from build123d import *

# Parameters (mm, degrees)
BOSS_EXTRUDE1_DEPTH     = 19.05
F_1_4_CLEARANCE_HOLE1_D = 6.5278
F_10_32_TAPPED_HOLE1_D  = 4.0386
SKETCH6_R               = 1.5875
CUT_EXTRUDE1_DEPTH      = 52.373383773
LPATTERN1_COUNT         = 9
LPATTERN1_PITCH         = 5.00126
FILLET1_R               = 3.429


with BuildPart() as part:
    # Sketch1 → Boss-Extrude1 (new body)
    with BuildSketch(Plane.XY):
        Polygon((0, 0), (17.3355, 0), (17.3355, 44.45), (0, 44.45), (0, 28.575), (9.525, 28.575), (9.525, 15.875), (0, 15.875), align=None)
    extrude(amount=BOSS_EXTRUDE1_DEPTH)

    # 1/4 Clearance Hole1 (through all)
    with Locations(Plane.XY.offset(19.05)):
        with Locations((5.842, 38.1), (5.842, 6.35)):
            Hole(F_1_4_CLEARANCE_HOLE1_D / 2)

    # #10-32 Tapped Hole1 (through all)
    with Locations(Plane(origin=(17.3355, 0, 0), x_dir=(0, 0, -1), z_dir=(1, 0, 0))):
        with Locations((-9.525, 14.605), (-9.525, 29.845)):
            Hole(F_10_32_TAPPED_HOLE1_D / 2)

    # Sketch6 → Cut-Extrude1 (cut, symmetric)
    with BuildSketch(Plane.XY.offset(19.05)):
        with Locations((17.018, 2.28092)):
            Circle(SKETCH6_R)
    cut_extrude1 = extrude(amount=CUT_EXTRUDE1_DEPTH, both=True, mode=Mode.SUBTRACT)

    # LPattern1: Cut-Extrude1 ×9
    with Locations(*[(0, i * LPATTERN1_PITCH, 0) for i in range(1, LPATTERN1_COUNT)]):
        add(cut_extrude1, mode=Mode.SUBTRACT)

    # Fillet1
    # the kernel refuses this fillet: 3.429 mm, written as the material it adds along each edge
    with BuildSketch(Plane(origin=(9.525, 15.875, 2.522427543), x_dir=(-1, 0, 0), z_dir=(0, 0, 1))) as fillet1_piece_1_section:
        with BuildLine():
            CenterArc((FILLET1_R, -FILLET1_R), FILLET1_R, 90, 90)
            Line((0, -FILLET1_R), (0, 0))
            Line((0, 0), (FILLET1_R, 0))
        make_face()
    fillet1_piece_1 = extrude(amount=16.527572457, mode=Mode.PRIVATE)
    fillet1_piece_1 = fillet1_piece_1 - Plane(origin=(8.790805855, 14.605, 9.525), x_dir=(0, 0, 1), z_dir=(-1, 0, 0)) * Cylinder(2.0193, 47, mode=Mode.PRIVATE)
    add(fillet1_piece_1)
    with BuildSketch(Plane(origin=(9.525, 28.575, 2.522427543), x_dir=(0, -1, 0), z_dir=(0, 0, 1))) as fillet1_piece_2_section:
        with BuildLine():
            CenterArc((FILLET1_R, -FILLET1_R), FILLET1_R, 90, 90)
            Line((0, -FILLET1_R), (0, 0))
            Line((0, 0), (FILLET1_R, 0))
        make_face()
    fillet1_piece_2 = extrude(amount=16.527572457, mode=Mode.PRIVATE)
    fillet1_piece_2 = fillet1_piece_2 - Plane(origin=(8.790805812, 29.845, 9.525), x_dir=(0, 0, 1), z_dir=(-1, 0, 0)) * Cylinder(2.0193, 47, mode=Mode.PRIVATE)
    add(fillet1_piece_2)
    with BuildSketch(Plane(origin=(9.525, 15.875, 0), x_dir=(-1, 0, 0), z_dir=(0, 0, 1))) as fillet1_piece_3_section:
        with BuildLine():
            CenterArc((FILLET1_R, -FILLET1_R), FILLET1_R, 90, 90)
            Line((0, -FILLET1_R), (0, 0))
            Line((0, 0), (FILLET1_R, 0))
        make_face()
    fillet1_piece_3 = extrude(amount=16.527572457, mode=Mode.PRIVATE)
    fillet1_piece_3 = fillet1_piece_3 - Plane(origin=(8.790805857, 14.605, 9.525), x_dir=(0, 0, 1), z_dir=(-1, 0, 0)) * Cylinder(2.0193, 47, mode=Mode.PRIVATE)
    add(fillet1_piece_3)
    with BuildSketch(Plane(origin=(9.525, 28.575, 0), x_dir=(0, -1, 0), z_dir=(0, 0, 1))) as fillet1_piece_4_section:
        with BuildLine():
            CenterArc((FILLET1_R, -FILLET1_R), FILLET1_R, 90, 90)
            Line((0, -FILLET1_R), (0, 0))
            Line((0, 0), (FILLET1_R, 0))
        make_face()
    fillet1_piece_4 = extrude(amount=16.527572457, mode=Mode.PRIVATE)
    fillet1_piece_4 = fillet1_piece_4 - Plane(origin=(8.790805811, 29.845, 9.525), x_dir=(0, 0, 1), z_dir=(-1, 0, 0)) * Cylinder(2.0193, 47, mode=Mode.PRIVATE)
    add(fillet1_piece_4)
    # the kernel refuses this fillet: 3.429 mm, written as the material it takes off along each edge
    with BuildSketch(Plane(origin=(0, 15.875, 2.522427543), x_dir=(1, 0, 0), z_dir=(0, 0, 1)), Plane(origin=(0, 15.875, -8.5725), x_dir=(1, 0, 0), z_dir=(0, 0, 1))) as fillet1_2_piece_1:
        with BuildLine():
            CenterArc((FILLET1_R, -FILLET1_R), FILLET1_R, 90, 90)
            Line((0, -FILLET1_R), (0, 0))
            Line((0, 0), (FILLET1_R, 0))
        make_face()
    extrude(amount=25.100072457, mode=Mode.SUBTRACT)
    with BuildSketch(Plane(origin=(0, 28.575, 2.522427543), x_dir=(1, 0, 0), z_dir=(0, 0, 1)), Plane(origin=(0, 28.575, -8.5725), x_dir=(1, 0, 0), z_dir=(0, 0, 1))) as fillet1_2_piece_2:
        with BuildLine():
            CenterArc((FILLET1_R, FILLET1_R), FILLET1_R, 180, 90)
            Line((0, FILLET1_R), (0, 0))
            Line((0, 0), (FILLET1_R, 0))
        make_face()
    extrude(amount=25.100072457, mode=Mode.SUBTRACT)
    with BuildSketch(Plane(origin=(0, 44.45, -8.5725), x_dir=(0, -1, 0), z_dir=(0, 0, 1)), Plane(origin=(0, 0, -8.5725), x_dir=(1, 0, 0), z_dir=(0, 0, 1))) as fillet1_2_piece_3:
        with BuildLine():
            CenterArc((FILLET1_R, FILLET1_R), FILLET1_R, 180, 90)
            Line((0, FILLET1_R), (0, 0))
            Line((0, 0), (FILLET1_R, 0))
        make_face()
    extrude(amount=36.195, mode=Mode.SUBTRACT)


solid = part.part
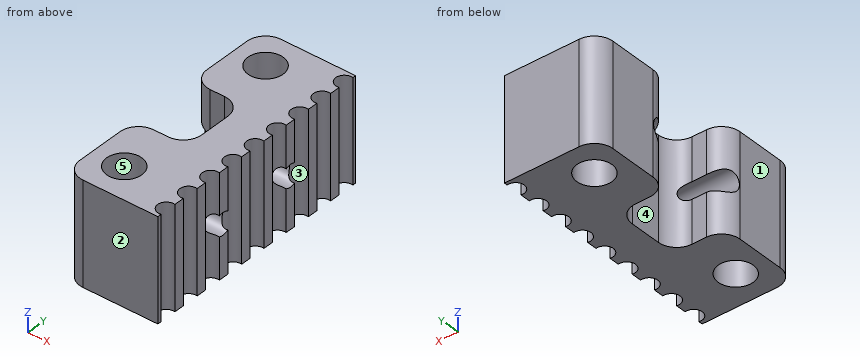
Here's how the part is built. I have some questions about the finished solid (model axes, mm). Face numbers are marked on the shaded views. A direction names the side the tool comes from. Round coordinates to 2 decimals unless told otherwise and drop trailing zeros. Write each loop counter-clockwise with the first axis right and the second up, starting at its lowest first coordinate (ties: lowest second). Pieces come first, ordered by that corner, then holes.
1. If we mould it in two halves opening along Y, with no side actions, what happens to the marked faces 1, 2 and 3? For each: released by +Y, released by -Y, zero draft, split by the parting line, or undercut.
2. Will these pins go through, and if not, where does the flat tip stop? pin 1 Ø3 at (y, z) = (23, 14) entering from -X (3 decimals); pin 2 Ø6 at (x, y) = (5.842, 38.1) entering from +Z; pin 3 Ø4 at (y, z) = (16, 16.5) entering from -X; pin 4 Ø6 at (y, z) = (27.5, 13) entering from -X.
3. Suppose I cut it at A-A (z = 4). State how many separate pieces and enclosed holes the cut face has, and give its area (3 significant figures).
4. Suppose I cut it at C-C (y = 38.1). List the corners of the cut face in (x, z) for me, and give its area (3 significant figures).
5. For the marked faces 4 and 5, which set-ups out of +Z, -Z, +X, -X, +Y, -Y let a thin tool reach every point of the face, with its end or its side?
6. Suppose I cut it at B-B (x = 8.5). List the corners of the cut face in (y, z) for me (3 decimals), and give its area (3 significant figures).
7. I need wall thicknesses on L1, parallel to Z at x = 6.75, y = 30; L2, parallel to Y at x = 5.5, z = 5.5 (3 decimals); L3, parallel to Y at x = 8.25, z = 16.25. Which ranges of each line are inside material? Lowest first, please.
Answer sheet:
1. face 1: zero draft
1. face 2: released by -Y
1. face 3: undercut
2. pin 1: stops at x = 9.525
2. pin 2: passes through
2. pin 3: stops at x = 0.37
2. pin 4: stops at x = 0.35
3. separate pieces: 1
3. enclosed holes: 2
3. area: 533 mm2
4. outline: (0, 0) - (2.58, 0) - (2.58, 19.05) - (0, 19.05) - close; (9.11, 0) - (15.65, 0) - (15.65, 19.05) - (9.11, 19.05) - close
4. area: 174 mm2
5. face 4: +Z, -Z, -X
5. face 5: +Z, -Z
6. outline: (0, 0) - (4.456, 0) - (4.456, 19.05) - (0, 19.05) - close; (8.244, 0) - (16.859, 0) - (16.859, 19.05) - (8.244, 19.05) - close; (27.591, 0) - (36.206, 0) - (36.206, 19.05) - (27.591, 19.05) - close; (39.994, 0) - (44.45, 0) - (44.45, 19.05) - (39.994, 19.05) - close; hole circle Ø4.039 at (14.605, 9.525); hole circle Ø4.039 at (29.845, 9.525)
6. area: 472 mm2
7. L1: z = 0 to 7.51, 11.54 to 19.05
7. L2: y = 0 to 3.104, 9.596 to 15.875, 28.575 to 34.854, 41.346 to 44.45
7. L3: y = 0 to 4.15, 8.55 to 16.64, 27.81 to 35.9, 40.3 to 44.45
